Check sheet for the modelled part. Datum: model origin and axes. Units: mm. A direction names the side the tool comes from. Round coordinates to 2 decimals unless told otherwise and drop trailing zeros. Loops run counter-clockwise (first coordinate to the right, second up) from the corner with the lowest first, then second, coordinate; pieces in that order, holes last. Notation, with made-up numbers: (45.25, -23.5) - (56.25, -23.5) arc R17 ccw to (56.25, 9.5) - close; hole circle Ø9 at (-32.75, -5). An arc over 180 degrees is marked (long way). Return JSON: item names as keys, results as strings.
Autodesk Inventor part; units mm, degrees
ref_plane "YZ Plane" through (0, 0, 0) normal (1, 0, 0) x (0, 1, 0)
ref_plane "XZ Plane" through (0, 0, 0) normal (0, 1, 0) x (-1, 0, 0)
ref_plane "XY Plane" through (0, 0, 0) normal (0, 0, 1) x (1, 0, 0)
sketch "Sketch1" plane through (0, 0, 0) normal (0, 0, 1) x (1, 0, 0)
  line L0 (34.925, -11.1125) -> (-34.925, -11.1125)
  line L1 (-34.925, -11.1125) -> (-34.925, 11.1125)
  line L2 (-34.925, 11.1125) -> (34.925, 11.1125)
  line L3 (34.925, 11.1125) -> (34.925, -11.1125)
  line L4 (34.925, -11.1125) -> (-34.925, 11.1125) construction
  line L5 (-34.925, -11.1125) -> (34.925, 11.1125) construction
  point P0 (0, 0)
  dimension "d0" = 69.85
  dimension "d1" = 22.225
extrude "Extrusion1" add sketch "Sketch1" along normal blind 79.375
sketch "Sketch2" plane through (0, 0, 79.375) normal (0, 0, 1) x (1, 0, 0)
  line L0 (23.606, -5.35) -> (-23.606, -5.35)
  line L1 (-28.956, 0) -> (-28.956, 0)
  line L2 (-23.606, 5.35) -> (23.606, 5.35)
  line L3 (28.956, 0) -> (28.956, 0)
  line L4 (28.956, -5.35) -> (-28.956, 5.35) construction
  line L5 (-28.956, -5.35) -> (28.956, 5.35) construction
  arc A0 (-23.606, 5.35) -> (-28.956, 0) centre (-23.606, 0) ccw
  arc A1 (-28.956, 0) -> (-23.606, -5.35) centre (-23.606, 0) ccw
  arc A2 (28.956, 0) -> (23.606, 5.35) centre (23.606, 0) ccw
  arc A3 (23.606, -5.35) -> (28.956, 0) centre (23.606, 0) ccw
  point P0 (0, 0)
  point P1 (28.956, 0)
  point P2 (-28.956, 0)
  dimension "d5" = 57.912
  dimension "d6" = 10.7
  dimension "d9" = 5.35
extrude "Extrusion2" cut sketch "Sketch2" against normal blind 69.85
fillet "Fillet1" radius 1.905 7 edges at (-34.925, 0, 79.375) (-34.925, 11.1125, 39.6875) (34.925, 0, 79.375) (34.925, 11.1125, 39.6875) (34.925, 0, 0) (0, 11.1125, 0) (-34.925, 0, 0)
sketch "Sketch3" plane through (0, 0, 0) normal (0, 0, -1) x (-1, 0, 0)
  line L0 (-23.606, -5.35) -> (23.606, -5.35)
  arc A0 (23.606, -5.35) -> (23.606, 5.35) centre (23.606, 0) ccw
  line L1 (23.606, 5.35) -> (-23.606, 5.35)
  arc A1 (-23.606, 5.35) -> (-23.606, -5.35) centre (-23.606, 0) ccw
  line L2 (6.5405, -2.1403) -> (-6.5405, -2.1403)
  line L3 (-6.5405, -2.1403) -> (-6.5405, 3.5747)
  line L4 (-6.5405, 3.5747) -> (6.5405, 3.5747)
  line L5 (6.5405, 3.5747) -> (6.5405, -2.1403)
  line L6 (6.5405, -2.1403) -> (-6.5405, 3.5747) construction
  line L7 (-6.5405, -2.1403) -> (6.5405, 3.5747) construction
  line L8 (33.02, 9.2075) -> (-33.02, 9.2075)
  line L9 (0, 9.2075) -> (0, -11.1125)
  line L10 (33.02, -11.1125) -> (-33.02, -11.1125)
  point P0 (0, 0)
  point P1 (0, 0.7172)
  dimension "d10" = 13.081
  dimension "d11" = 5.715
  dimension "d13" = 4.6328
extrude "Extrusion3" cut sketch "Sketch3" against normal through all contours L9 L4 L5 L2 | L2 L3 L4 L9
sketch "Sketch5" plane through (-33.02, 11.1125, 79.375) normal (0, 1, 0) x (1, 0, 0)
  line L0 (33.02, 79.375) -> (33.02, 0)
  line L1 (20.32, 0) -> (20.32, 19.05)
  line L2 (20.32, 19.05) -> (33.02, 19.05)
  line L3 (20.32, 0) -> (33.02, 0)
  line L4 (66.04, 0) -> (0, 0)
  line L5 (45.72, 0) -> (45.72, 19.05)
  line L6 (45.72, 19.05) -> (33.02, 19.05)
  line L7 (45.72, 0) -> (33.02, 0)
  point P0 (33.02, 0)
  point P1 (45.72, 0)
  dimension "d22" = 19.05
  dimension "d23" = 12.7
extrude "Extrusion5" cut sketch "Sketch5" against normal through all
fillet "Fillet3" radius 1.905 18 edges at (-34.367, 10.5545, 78.817) (-22.86, 11.1125, 79.375) (-12.7, 11.1125, 69.85) (0, 11.1125, 60.325) (12.7, 11.1125, 69.85) (12.7, 8.2313, 79.375) (0, -5.35, 60.325) (-12.7, -5.35, 69.85) (12.7, -5.35, 69.85) (12.7, -8.2313, 79.375) (-12.7, -8.2313, 79.375) (34.367, 10.5545, 78.817) (22.86, 11.1125, 79.375) (-12.7, 8.2312, 79.375) (-12.7, 8.2312, 60.325) (12.7, -8.2313, 60.325) (12.7, 8.2313, 60.325) (-12.7, -8.2313, 60.325)
properties part number "_3DPrint"
Q1. Draft check along Y on faces 1 (the face through (-23.94, 10.54, 78.83)), 2 (the face through (-6.54, 1, 5)), 3 (the face through (0, -11.112, 39)), 4 (the face through (0, 7, 60.325)). Enter one of: released by +Y, released by -Y, zero draft, split by the parting line, or undercut.
Answer key:
{"face 1": "released by +Y", "face 2": "undercut", "face 3": "released by -Y", "face 4": "zero draft"}
Q2. Sectioned sample at A-A (y = 0). Enter the section's corners in (x, z) (1 decimal), plus the area to 3 significant figures.
Answer key:
{"outline": "(-34.9, 1.9) arc R1.9 ccw to (-33, 0) - (-6.5, 0) - (-6.5, 9.5) - (-29, 9.5) - (-29, 79.4) - (-33, 79.4) arc R1.9 ccw to (-34.9, 77.5) - close; (6.5, 0) - (33, 0) arc R1.9 ccw to (34.9, 1.9) - (34.9, 77.5) arc R1.9 ccw to (33, 79.4) - (29, 79.4) - (29, 9.5) - (6.5, 9.5) - close", "area": "1,370 mm²"}
Q3. Tool access check on faces 5 (the face through (13.273, 10.569, 69.957)), 6 (the face through (0, 3.575, 5)), 7 (the face through (13.273, -5.893, 70.923)). Record the directions out of +Z, -Z, +X, -X, +Y, -Y that give a thin tool (end or side, any length) a straight path to the whole face; none if there is none.
Answer key:
{"face 5": "+Z, +Y", "face 6": "+Z, -Z", "face 7": "+Z"}
Q4. Scan lines: probe 1 along X at (y, z) = (-2, 9) (1 decimal); probe 2 along Y at (x, z) = (2, 37.5); probe 3 along Z at (x, y) = (-7.5, -3.5) (3 decimals). Record each from-to range of solid material in increasing order. Write a range as [from, to].
Answer key:
{"probe 1": "x = [-34.9, -6.5], [6.5, 34.9]", "probe 2": "y = [-11.11, -5.35], [5.35, 11.11]", "probe 3": "z = [0, 9.525]"}
Q5. Depth check by flat-ended pin: P1, Ø4, axis at x = 3.5, y = -9, coming from the +Z side (3 decimals); P2, Ø10, axis at x = 9, y = -6, coming from the +Z side; P3, Ø3, axis at x = 1, y = -2, coming from the +Z side (3 decimals). Enter the tip coordinate at first touch or a pass-through.
Answer key:
{"P1": "stops at z = 60.325", "P2": "stops at z = 79.28", "P3": "stops at z = 9.525"}
